For this review, take the finished solid that the model builds, in its own axes (mm). A direction names the side the tool comes from. Round coordinates to 2 decimals unless told otherwise and drop trailing zeros. Loops run counter-clockwise (first coordinate to the right, second up) from the corner with the lowest first, then second, coordinate; pieces in that order, holes last.
```python
from build123d import *

# Parameters (mm, degrees)
F0_W     = 88.9
F0_H     = 76.2
F1_DEPTH = 88.9
F2_R     = 34.925
F3_DEPTH = 25.4
F4_R     = 38.989
F5_DEPTH = 50.8
F6_W     = 6.35
F6_H     = 6.35
F7_DEPTH = 2.54
F8_R     = 3.556
F9_DEPTH = 12.7
F10_R    = 31.75


with BuildPart() as f1:
    # F0 (on Right) → F1 (new body)
    with BuildSketch(Plane.YZ):
        with Locations((-44.45, 38.1)):
            Rectangle(F0_W, F0_H)
        Polygon((0, 76.2), (0, 0), (6.35, 0), (26.7677284633, 76.2), align=None)
    extrude(amount=F1_DEPTH)

    # F2 (on face) → F3 (cut)
    with BuildSketch(Plane(origin=(0, 0, 0), x_dir=(1, 0, 0), z_dir=(0, 0, -1))):
        with Locations((44.45, 41.275)):
            Circle(F2_R)
    extrude(amount=-F3_DEPTH, mode=Mode.SUBTRACT)

    # F4 (on face) → F5 (cut)
    with BuildSketch(Plane.XY.offset(76.2)):
        with Locations((44.45, -41.275)):
            Circle(F4_R)
    extrude(amount=-F5_DEPTH, mode=Mode.SUBTRACT)

    # F6 (on face) → F7 (join)
    with BuildSketch(Plane(origin=(0, 0, 0), x_dir=(1, 0, 0), z_dir=(0, 0, -1))):
        with BuildLine():
            Line((79.2303824016, 44.45), (47.625, 44.45))
            Line((47.625, 44.45), (47.625, 38.1))
            Line((47.625, 38.1), (79.2303824016, 38.1))
            ThreePointArc((79.2303824016, 38.1), (79.3388268675, 39.6858540619), (79.375, 41.275))
            ThreePointArc((79.375, 41.275), (79.3388268675, 42.8641459381), (79.2303824016, 44.45))
        make_face()
        with BuildLine():
            Line((41.275, 76.0553824016), (41.275, 44.45))
            Line((41.275, 44.45), (47.625, 44.45))
            Line((47.625, 44.45), (47.625, 76.0553824016))
            ThreePointArc((47.625, 76.0553824016), (44.45, 76.2), (41.275, 76.0553824016))
        make_face()
        with BuildLine():
            Line((41.275, 44.45), (9.6696175984, 44.45))
            ThreePointArc((9.6696175984, 44.45), (9.525, 41.275), (9.6696175984, 38.1))
            Line((9.6696175984, 38.1), (41.275, 38.1))
            Line((41.275, 38.1), (41.275, 44.45))
        make_face()
        with Locations((44.45, 41.275)):
            Rectangle(F6_W, F6_H)
        with BuildLine():
            Line((47.625, 38.1), (41.275, 38.1))
            Line((41.275, 38.1), (41.275, 6.4946175984))
            ThreePointArc((41.275, 6.4946175984), (44.45, 6.35), (47.625, 6.4946175984))
            Line((47.625, 6.4946175984), (47.625, 38.1))
        make_face()
    extrude(amount=-F7_DEPTH)

    # F8 (on face) → F9 (cut)
    with BuildSketch(Plane(origin=(0, 5.924630657, -1.5875), x_dir=(-1, 0, 0), z_dir=(0, 0.9659258263, -0.2588190451))):
        with Locations((-69.85, 66.48752341)):
            Circle(F8_R)
        with Locations((-19.05, 66.48752341)):
            Circle(F8_R)
        with Locations((-69.85, 15.68752341)):
            Circle(F8_R)
        with Locations((-19.05, 15.68752341)):
            Circle(F8_R)
    extrude(amount=-F9_DEPTH, mode=Mode.SUBTRACT)

    # F10
    f10_edges = [f1.edges().sort_by_distance(p)[0] for p in [
        (0, -88.9, 38.1),
        (88.9, -88.9, 38.1),
    ]]
    fillet(f10_edges, radius=F10_R)


solid = f1.part
```
(1) For L1, parallel to Y at x = 79, z = 47.5; L2, parallel to X at y = -62, z = 43; L3, parallel to X at y = -17.5, z = 66, list the stretches that pass through material, from the lowest coordinate up.
(2) Insertion check: pin 1 Ø2 at (x, z) = (69, 1) entering from -Y; pin 2 Ø4 at (x, z) = (69, 60) entering from +Y; pin 3 Ø5 at (x, y) = (32, -9) entering from +Z. Each pin has a flat end and moves straight along its axis. Give the tip position at first contact, or say it passes through.
(3) The part is to be moulded in two halves that separate along Z. For faces 1 (the flat face through (24, -5, 76.2)), 2 (the flat face through (0, -25, 39)), 3 (the flat face through (69.9, 10.88, 65.97)), say which applies: pulls with the +Z half, pulls with the -Z half, needs draft (parallel to the pull), parting line crosses it, or undercut.
(4) Add section B-B (y = -16). Give the boundary of the cut face in (x, z) (3 decimals), plus the area to 3 significant figures.
(5) For faces 4 (the flat face through (44, -42, 0)), 5 (the flat face through (69.9, -2.27, 16.9)), 6 (the flat face through (41.275, -60, 1)), 7 (the flat face through (15, -61, 25.4)), list the 3-axis set-ups (+Z, -Z, +X, -X, +Y, -Y) from which the entire face can be reached by the end or side of a thin tool; tool diameter is ignored.
(6) Add section A-A (x = 38.5). Give the boundary of the cut face in (y, z), plus the area to 3 significant figures.
(7) Add section D-D (z = 32). Give the boundary of the cut face in (x, y) (3 decimals).
(8) Add section C-C (z = 71). Give the boundary of the cut face in (x, y) (3 decimals).
Outcome:
1. L1: y = -80.19 to -59.34, -23.21 to 19.08
1. L2: x = 0.37 to 11.43, 77.47 to 88.53
1. L3: x = 0 to 13.55, 75.35 to 88.9
2. pin 1: stops at y = -86.99
2. pin 2: stops at y = 22.56
2. pin 3: stops at z = 25.4
3. face 1: pulls with the +Z half
3. face 2: needs draft
3. face 3: undercut
4. outline: (0, 0) - (20.348, 0) - (20.348, 25.4) - (14.763, 25.4) - (14.763, 76.2) - (0, 76.2) - close; (41.275, 0) - (47.625, 0) - (47.625, 2.54) - (41.275, 2.54) - close; (68.552, 0) - (88.9, 0) - (88.9, 76.2) - (74.137, 76.2) - (74.137, 25.4) - (68.552, 25.4) - close
4. area: 2,550 mm2
5. face 4: -Z, +X, -X, +Y, -Y
5. face 5: none
5. face 6: +Z, -Z
5. face 7: +Z
6. outline: (-88.9, 0) - (-75.69, 0) - (-75.69, 25.4) - (-79.81, 25.4) - (-79.81, 76.2) - (-88.9, 76.2) - close; (-44.45, 0) - (-38.1, 0) - (-38.1, 2.54) - (-44.45, 2.54) - close; (-6.86, 0) - (6.35, 0) - (26.77, 76.2) - (-2.74, 76.2) - (-2.74, 25.4) - (-6.86, 25.4) - close
6. area: 2,390 mm2
7. outline: (0, -57.15) arc R31.75 ccw to (31.75, -88.9) - (57.15, -88.9) arc R31.75 ccw to (88.9, -57.15) - (88.9, 14.924) - (0, 14.924) - close; hole circle Ø77.978 at (44.45, -41.275)
8. outline: (0, -57.15) arc R31.75 ccw to (31.75, -88.9) - (57.15, -88.9) arc R31.75 ccw to (88.9, -57.15) - (88.9, 25.374) - (0, 25.374) - close; hole circle Ø77.978 at (44.45, -41.275)
